Geometry check sheet. Reference: the model listing, model coordinates, mm. Face numbers are marked on the shaded views. A direction names the side the tool comes from. Give positions to 0.01 mm unless a question says otherwise; leave off trailing zeros. Write each loop counter-clockwise with the first axis right and the second up, starting at its lowest first coordinate (ties: lowest second). Pieces come first, ordered by that corner, then holes. Notation, with made-up numbers: M 20.5,6.25 L 63.5,6.25 A22 cw 63.5,39.25 Z; hole C 16,77.25 d9. An arc over 180 degrees is marked long. Write each question's results on one line, items separated by ' | '.
```python
from build123d import *

# Parameters (mm, degrees)
ESTRUSIONE_ESTRUSIONE1_DEPTH = 7
SCHIZZO2_R                   = 0.9
TAGLIO_ESTRUSIONE1_DEPTH     = 21.420394218
TAGLIO_ESTRUSIONE2_REACH     = 37.195
SCHIZZO3_R                   = 1.4


with BuildPart() as part:
    # Schizzo1 → Estrusione-Estrusione1 (new body)
    with BuildSketch(Plane.XY):
        Polygon((8.3, 11.55), (-4, 11.55), (-4, -11.55), (8.3, -11.55), (8.3, -16.55), (-9.7, -16.55), (-9.7, 16.55), (8.3, 16.55), align=None)
    extrude(amount=ESTRUSIONE_ESTRUSIONE1_DEPTH)

    # Schizzo2 → Taglio-Estrusione1 (cut, through all)
    with BuildSketch(Plane.XY.offset(7)):
        with Locations((2.6, 14.05)):
            Circle(SCHIZZO2_R)
        with Locations(Location((2.6, -14.05, 0), (0, 0, 180))):
            Circle(SCHIZZO2_R)
    extrude(amount=-TAGLIO_ESTRUSIONE1_DEPTH, mode=Mode.SUBTRACT)

    # Schizzo3 → Taglio-Estrusione2 (cut, up to next)
    with BuildSketch(Plane.XZ.offset(16.55), mode=Mode.PRIVATE) as taglio_estrusione2_sk1:
        with Locations(Location((-0.7, 3.5, 0), (0, 0, 270))):
            Circle(SCHIZZO3_R)
    taglio_estrusione2_tool1 = extrude(taglio_estrusione2_sk1.sketch, amount=-TAGLIO_ESTRUSIONE2_REACH, mode=Mode.PRIVATE) & part.part
    add(taglio_estrusione2_tool1.solids().sort_by_distance((-0.7, -16.55, 3.5))[0], mode=Mode.SUBTRACT)


solid = part.part
```
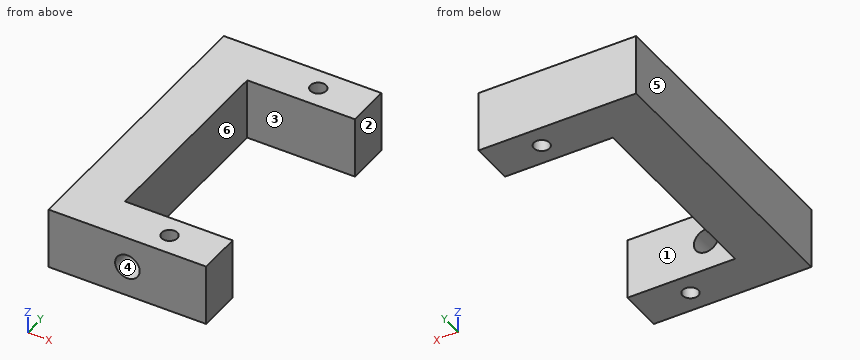
Q1. Material ranges on probe 1 along Y at (x, z) = (2.6, 1.5); probe 2 along X at (y, z) = (-14.05, 5.25); probe 3 along X at (y, z) = (-15.15, 3.5), recorded low to high. Write a range as [from, to].
Answer key:
probe 1: y = [-16.55, -14.95], [-13.15, -11.55], [11.55, 13.15], [14.95, 16.55] | probe 2: x = [-9.7, 1.7], [3.5, 8.3] | probe 3: x = [-9.7, -2.1], [0.7, 8.3]
Q2. Section check B-B (x = -0.7). Enter the section's corners in (y, z), then the cut area to 3 significant figures.
Answer key:
outline: M -16.55,0 L -11.55,0 L -11.55,2.1 L -16.55,2.1 Z; M -16.55,4.9 L -11.55,4.9 L -11.55,7 L -16.55,7 Z; M 11.55,0 L 16.55,0 L 16.55,7 L 11.55,7 Z | area: 56.0 mm2
Q3. Section check D-D (x = -2.75). Enter the section's corners in (y, z), then the cut area to 3 significant figures.
Answer key:
outline: M -16.55,0 L -11.55,0 L -11.55,7 L -16.55,7 Z; M 11.55,0 L 16.55,0 L 16.55,7 L 11.55,7 Z | area: 70.0 mm2
Q4. Release check for a two-part mould opening along X. For the marked faces 3, 4, 5 and 6 record: released by +X, released by -X, zero draft, split by the parting line, or undercut.
Answer key:
face 3: zero draft | face 4: undercut | face 5: released by -X | face 6: released by +X
Q5. Section check A-A (z = 3.5). Enter the section's corners in (x, y).
Answer key:
outline: M -9.7,-16.55 L -2.1,-16.55 L -2.1,-11.55 L -4,-11.55 L -4,11.55 L 8.3,11.55 L 8.3,16.55 L -9.7,16.55 Z; M 0.7,-16.55 L 8.3,-16.55 L 8.3,-11.55 L 0.7,-11.55 Z; hole C 2.6,-14.05 d1.8; hole C 2.6,14.05 d1.8
Q6. Access from +Z, -Z, +X, -X, +Y, -Y to the whole of each face (thin tool, end or side, straight path). Record for the marked faces 1 and 2.
Answer key:
face 1: +Z, -Z, +X | face 2: +Z, -Z, +X, +Y, -Y
Q7. Section check C-C (y = -14.05). Enter the section's corners in (x, z), then the cut area to 3 significant figures.
Answer key:
outline: M -9.7,0 L 1.7,0 L 1.7,7 L -9.7,7 Z; M 3.5,0 L 8.3,0 L 8.3,7 L 3.5,7 Z; hole C -0.7,3.5 d2.8 | area: 107 mm2
Q8. Depth check by flat-ended pin: P1, Ø2, axis at x = -0.7, z = 3.5, coming from the -Y side. Enter the tip coordinate at first touch or a pass-through.
Answer key:
P1: stops at y = 11.55
